Here's how the part is built. I have some questions about the finished solid (model axes, mm). A direction names the side the tool comes from. Round coordinates to 2 decimals unless told otherwise and drop trailing zeros. Write each loop counter-clockwise with the first axis right and the second up, starting at its lowest first coordinate (ties: lowest second). Pieces come first, ordered by that corner, then holes. Notation, with made-up numbers: M -21.75,-5 L 34.25,-5 A19 ccw 34.25,3 Z; hole C -31.5,63 d4. An arc over 180 degrees is marked long. Write item = value, one per line. Start each with the question number.
(1) On a 3-axis mill with a long thin cutter (end or side, diameter ignored), from which of +Z, -Z, +X, -X, +Y, -Y can I reach the whole of each face in a straight line? I mean faces 1 (the cylindrical face through (-2.685, -0.596, -1.56)), 2 (the flat face through (-0.616, 1.088, -0.641)), 3 (the flat face through (-1, -2, -3)). Say none if no direction works.
(2) I want a section at A-A (z = -12.5). List the corners of the cut face in (x, y) for me, and give its area (3 significant figures).
(3) If we mould it in two halves opening along X, with no side actions, what happens to faces 4 (the conical face through (0.06, 0.19, -1.906)), 5 (the flat face through (0, 0, -23)), 6 (the cylindrical face through (0.07, -1.5, -13.26))? For each: released by +X, released by -X, zero draft, split by the parting line, or undercut.
(4) I need wall thicknesses on line 1 along Z through (x, y) = (-2, -0.95); line 2 along Y through (x, z) = (0.45, -1.25); line 3 along X through (y, z) = (0, -20). Which ranges of each line are inside material? Lowest first, please.
(5) Will this pin go through, and if not, where does the flat tip stop? pin 1 Ø2 at (y, z) = (0.5, -2.5) entering from -X.
```python
from build123d import *

# Parameters (mm, degrees)
CUT_EXTRUDE1_DEPTH = 1.3


with BuildPart() as part:
    # Sketch1 → Revolve1 (revolve)
    with BuildSketch(Plane(origin=(0, 0, 0), x_dir=(0, 0, -1), z_dir=(1, 0, 0))):
        with BuildLine():
            Line((0, 0), (0, 2.45))
            Line((0, 2.45), (0.3, 2.75))
            Line((0.3, 2.75), (2.785, 2.75))
            Line((2.785, 2.75), (3, 2.535))
            Line((3, 2.535), (3, 1.8))
            ThreePointArc((3, 1.8), (3.015193643, 1.74701055), (3.056157637, 1.710123155))
            Line((3.056157637, 1.710123155), (3.466157637, 1.510123155))
            ThreePointArc((3.466157637, 1.510123155), (3.48750205, 1.50256365), (3.51, 1.5))
            Line((3.51, 1.5), (22.75, 1.5))
            Line((22.75, 1.5), (23, 1.25))
            Line((23, 1.25), (23, 0))
            Line((23, 0), (0, 0))
        make_face()
    revolve(axis=Axis((0, 0, 0), (0, 0, -1)))

    # Sketch2 → Cut-Extrude1 (cut)
    with BuildSketch(Plane.XY):
        Polygon((0, 1.443375673), (-1.25, 0.721687836), (-1.25, -0.721687836), (0, -1.443375673), (1.25, -0.721687836), (1.25, 0.721687836), align=None)
    extrude(amount=-CUT_EXTRUDE1_DEPTH, mode=Mode.SUBTRACT)

    # Sketch3 → Cut-Revolve2 (revolve, cut)
    with BuildSketch(Plane(origin=(0, 0, 0), x_dir=(0, 0, -1), z_dir=(1, 0, 0))):
        Polygon((1.3, 0), (1.3, 1.25), (2.021687836, 0), align=None)
    revolve(axis=Axis((0, 0, -1.3), (0, 0, -1)), mode=Mode.SUBTRACT)

    # Sketch4 → Cut-Revolve3 (revolve, cut)
    with BuildSketch(Plane(origin=(0, 0, 0), x_dir=(0, 0, -1), z_dir=(1, 0, 0))):
        Polygon((0, 1.443375673), (0, 1.25), (0.051814855, 1.25), align=None)
    revolve(axis=Axis((0, 0, 0), (0, 0, -1)), mode=Mode.SUBTRACT)


solid = part.part
```
Returned:
q1.face_1 = +Z, -Z
q1.face_2 = +Z
q1.face_3 = -Z
q2.outline = C 0,0 d3
q2.area = 7.07 mm²
q3.face_4 = undercut
q3.face_5 = zero draft
q3.face_6 = split by the parting line
q4.line_1 = -3 to 0
q4.line_2 = -2.71 to -1.18, 1.18 to 2.71
q4.line_3 = -1.5 to 1.5
q5.pin_1 = -2.75
